from build123d import *

# Parameters (mm, degrees)
EXTRUDE_1_DEPTH     = 25
CUT_EXTRUDE_1_REACH = 77.67
SKETCH_2_R          = 11
SKETCH_2_R_2        = 1.75
CUT_EXTRUDE_2_REACH = 77.75
CHAMFER_1_SIZE      = 5
FILLET_1_R          = 2
EXTRUDE_2_DEPTH     = 2.5


with BuildPart() as part:
    # 草图1 → 凸台-拉伸1 (new, symmetric)
    with BuildSketch(Plane.XY):
        Polygon((0, 0), (-53, 0), (-53, 51), (-50, 51), (-50, 3), (0, 3), align=None)
    extrude(amount=EXTRUDE_1_DEPTH, both=True)

    # 草图2 → 切除-拉伸1 (cut, up to next)
    with BuildSketch(Plane(origin=(-50, 0, 0), x_dir=(0, 0, -1), z_dir=(1, 0, 0)), mode=Mode.PRIVATE) as cut_extrude_1_sk1:
        with Locations(Location((0, 30, 0), (0, 0, 90))):
            Circle(SKETCH_2_R)
    cut_extrude_1_tool1 = extrude(cut_extrude_1_sk1.sketch, amount=-CUT_EXTRUDE_1_REACH, mode=Mode.PRIVATE) & part.part
    # 草图2 → 切除-拉伸1 (cut, up to next)
    with BuildSketch(Plane(origin=(-50, 0, 0), x_dir=(0, 0, -1), z_dir=(1, 0, 0)), mode=Mode.PRIVATE) as cut_extrude_1_sk2:
        with Locations(Location((-15.5, 45.5, 0), (0, 0, 90))):
            Circle(SKETCH_2_R_2)
    cut_extrude_1_tool2 = extrude(cut_extrude_1_sk2.sketch, amount=-CUT_EXTRUDE_1_REACH, mode=Mode.PRIVATE) & part.part
    # 草图2 → 切除-拉伸1 (cut, up to next)
    with BuildSketch(Plane(origin=(-50, 0, 0), x_dir=(0, 0, -1), z_dir=(1, 0, 0)), mode=Mode.PRIVATE) as cut_extrude_1_sk3:
        with Locations(Location((15.5, 45.5, 0), (0, 0, 90))):
            Circle(SKETCH_2_R_2)
    cut_extrude_1_tool3 = extrude(cut_extrude_1_sk3.sketch, amount=-CUT_EXTRUDE_1_REACH, mode=Mode.PRIVATE) & part.part
    # 草图2 → 切除-拉伸1 (cut, up to next)
    with BuildSketch(Plane(origin=(-50, 0, 0), x_dir=(0, 0, -1), z_dir=(1, 0, 0)), mode=Mode.PRIVATE) as cut_extrude_1_sk4:
        with Locations(Location((-15.5, 14.5, 0), (0, 0, 90))):
            Circle(SKETCH_2_R_2)
    cut_extrude_1_tool4 = extrude(cut_extrude_1_sk4.sketch, amount=-CUT_EXTRUDE_1_REACH, mode=Mode.PRIVATE) & part.part
    # 草图2 → 切除-拉伸1 (cut, up to next)
    with BuildSketch(Plane(origin=(-50, 0, 0), x_dir=(0, 0, -1), z_dir=(1, 0, 0)), mode=Mode.PRIVATE) as cut_extrude_1_sk5:
        with Locations(Location((15.5, 14.5, 0), (0, 0, 90))):
            Circle(SKETCH_2_R_2)
    cut_extrude_1_tool5 = extrude(cut_extrude_1_sk5.sketch, amount=-CUT_EXTRUDE_1_REACH, mode=Mode.PRIVATE) & part.part
    add(cut_extrude_1_tool1.solids().sort_by_distance((-50, 30, 0))[0], mode=Mode.SUBTRACT)
    add(cut_extrude_1_tool2.solids().sort_by_distance((-50, 45.5, 15.5))[0], mode=Mode.SUBTRACT)
    add(cut_extrude_1_tool3.solids().sort_by_distance((-50, 45.5, -15.5))[0], mode=Mode.SUBTRACT)
    add(cut_extrude_1_tool4.solids().sort_by_distance((-50, 14.5, 15.5))[0], mode=Mode.SUBTRACT)
    add(cut_extrude_1_tool5.solids().sort_by_distance((-50, 14.5, -15.5))[0], mode=Mode.SUBTRACT)

    # 草图3 → 切除-拉伸2 (cut, up to next)
    with BuildSketch(Plane(origin=(0, 3, 0), x_dir=(1, 0, 0), z_dir=(0, 1, 0)), mode=Mode.PRIVATE) as cut_extrude_2_sk1:
        with BuildLine():
            Line((-41, 17.1), (-11, 17.1))
            ThreePointArc((-11, 17.1), (-8.9, 15), (-11, 12.9))
            Line((-11, 12.9), (-41, 12.9))
            ThreePointArc((-41, 12.9), (-43.1, 15), (-41, 17.1))
        make_face()
    cut_extrude_2_tool1 = extrude(cut_extrude_2_sk1.sketch, amount=-CUT_EXTRUDE_2_REACH, mode=Mode.PRIVATE) & part.part
    # 草图3 → 切除-拉伸2 (cut, up to next)
    with BuildSketch(Plane(origin=(0, 3, 0), x_dir=(1, 0, 0), z_dir=(0, 1, 0)), mode=Mode.PRIVATE) as cut_extrude_2_sk2:
        with BuildLine():
            Line((-41, -12.9), (-11, -12.9))
            ThreePointArc((-11, -12.9), (-8.9, -15), (-11, -17.1))
            Line((-11, -17.1), (-41, -17.1))
            ThreePointArc((-41, -17.1), (-43.1, -15), (-41, -12.9))
        make_face()
    cut_extrude_2_tool2 = extrude(cut_extrude_2_sk2.sketch, amount=-CUT_EXTRUDE_2_REACH, mode=Mode.PRIVATE) & part.part
    add(cut_extrude_2_tool1.solids().sort_by_distance((-26, 3, -15))[0], mode=Mode.SUBTRACT)
    add(cut_extrude_2_tool2.solids().sort_by_distance((-26, 3, 15))[0], mode=Mode.SUBTRACT)

    # 倒角1
    chamfer_1_edges = [part.edges().sort_by_distance(p)[0] for p in [
        (-51.5, 51, 25),
        (0, 1.5, 25),
        (-51.5, 51, -25),
        (0, 1.5, -25),
    ]]
    chamfer(chamfer_1_edges, length=CHAMFER_1_SIZE)

    # 圆角1
    fillet_1_edges = [part.edges().sort_by_distance(p)[0] for p in [
        (-53, 0, 0),
        (-50, 3, 0),
    ]]
    fillet(fillet_1_edges, radius=FILLET_1_R)

    # 草图4 → 凸台-拉伸2 (add)
    with BuildSketch(Plane.XY.offset(25)):
        Polygon((-50, 23), (-50, 5), (-48, 3), (-37, 3), align=None)
    extrude_2 = extrude(amount=-EXTRUDE_2_DEPTH)

    # 镜向1: 凸台-拉伸2 across plane
    add(extrude_2.mirror(Plane.XY))


solid = part.part
Could you check a few things on this model? Use its own coordinates, in mm. A direction names the side the tool comes from. Round coordinates to 2 decimals unless told otherwise and drop trailing zeros. Order: outer loops, then holes, each group sorted by start corner. A loop starts at its lowest first (then second) coordinate and runs counter-clockwise, first axis right, second up.
Q1. Imagine slicing it at D-D, the plane z = -12. List the corners of the cut face in (x, y) for me, then the cut area to 3 significant figures.
Geometry says:
outline: (-53, 2) arc R2 ccw to (-51, 0) - (0, 0) - (0, 3) - (-48, 3) arc R2 cw to (-50, 5) - (-50, 51) - (-53, 51) - close
area: 303 mm2
Q2. Please list where these lines run through material, in increasing order: probe 1 along Z at (x, y) = (-51.15, 14.5); probe 2 along Z at (x, y) = (-49.5, 22); probe 3 along Z at (x, y) = (-51, 30).
Geometry says:
probe 1: z = -25 to -17.25, -13.75 to 13.75, 17.25 to 25
probe 2: z = -25 to -22.5, 22.5 to 25
probe 3: z = -25 to -11, 11 to 25
Q3. Imagine slicing it at A-A, the plane x = -27.5. List the corners of the cut face in (y, z) for me.
Geometry says:
outline: (0, -25) - (3, -25) - (3, -17.1) - (0, -17.1) - close; (0, -12.9) - (3, -12.9) - (3, 12.9) - (0, 12.9) - close; (0, 17.1) - (3, 17.1) - (3, 25) - (0, 25) - close
Q4. I'm going to push flat-ended pins straight in: P1, Ø3, axis at y = 14.5, z = 15.5, coming from the +X side; P2, Ø14.5, axis at x = -29.5, z = 8.5, coming from the +Y side; P3, Ø4, axis at y = 13.5, z = 12.5, coming from the +X side. Where does each tip first touch, or does it pass through?
Geometry says:
P1: passes through
P2: stops at y = 3
P3: stops at x = -50
Q5. Imagine slicing it at C-C, the plane z = 0. List the corners of the cut face in (x, y) for me, then the cut area to 3 significant figures.
Geometry says:
outline: (-53, 2) arc R2 ccw to (-51, 0) - (0, 0) - (0, 3) - (-48, 3) arc R2 cw to (-50, 5) - (-50, 19) - (-53, 19) - close; (-53, 41) - (-50, 41) - (-50, 51) - (-53, 51) - close
area: 237 mm2
Q6. Thinking about a two-plate mould opening in Z: for faces 4 (the face through (-42, 9, -25)), 5 (the face through (-51.479, 47.169, -14.974)), 6 (the face through (-43.41, 12.86, 23.77)), which applies, released by +Z, released by -Z, zero draft, split by the parting line, or undercut?
Geometry says:
face 4: released by -Z
face 5: undercut
face 6: zero draft
Q7. Which directions (+Z, -Z, +X, -X, +Y, -Y) give clear straight access to the entire face, cutting with the end or side of a thin tool? Please do faces 1 (the face through (-50, 18, 0)), 2 (the face through (-51.479, 14.272, 17.235)), 3 (the face through (-26, 2, -12.9)).
Geometry says:
face 1: +X, +Y
face 2: +X, -X
face 3: +Y, -Y
Q8. Imagine slicing it at B-B, the plane y = 30. List the corners of the cut face in (x, z) for me.
Geometry says:
outline: (-53, -25) - (-50, -25) - (-50, -11) - (-53, -11) - close; (-53, 11) - (-50, 11) - (-50, 25) - (-53, 25) - close
